Answer from the drawing. Dimensions are ordinates in mm from the lowest x, y and z of the part. Give positions to 0.01 mm unless a question says otherwise; leave off trailing zeros. One line per item, written item: value.
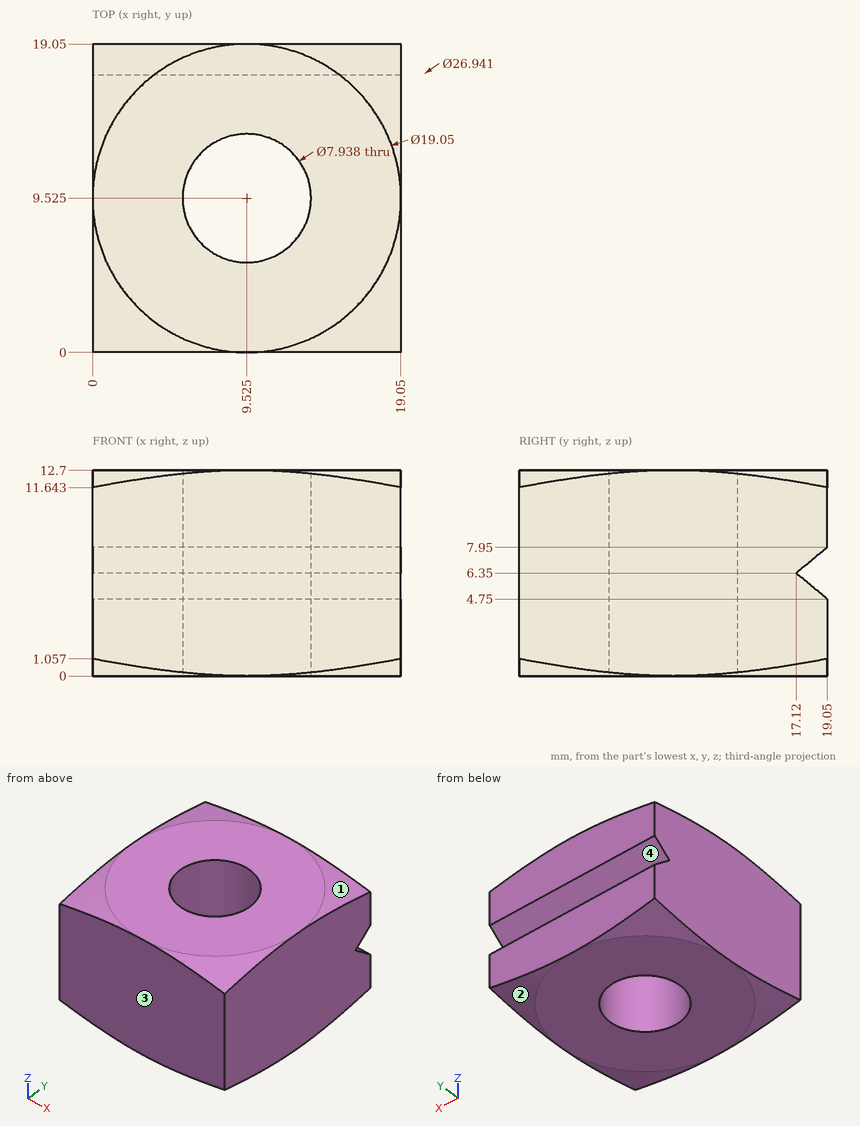
(1) Given P1, Ø7, axis at x = 9.525, y = 9.525, coming from the -Z side, flat-ended and moving along its own axis, determine where the tip first touches the part or whether it passes through.
Findings:
P1: passes through
(2) Find the intervals of material crossed by probe 1 along Y at (x, z) = (9.5, 9.5); probe 2 along X at (y, z) = (12.25, 2); probe 3 along Y at (x, z) = (8.75, 11), in increasing order. Write a range as from..to.
Findings:
probe 1: y = 0..5.56, 13.49..19.05
probe 2: x = 0..6.64, 12.41..19.05
probe 3: y = 0..5.63, 13.42..19.05
(3) Determine the mould class of the marked faces 1, 2, 3 and 4 for opening direction Z: pulls with the +Z half, pulls with the -Z half, needs draft (parallel to the pull), parting line crosses it, or undercut.
Findings:
face 1: pulls with the +Z half
face 2: pulls with the -Z half
face 3: needs draft
face 4: undercut
